Can you work these out from the model? Positions are in its coordinate system, mm. A direction names the side the tool comes from. Give positions to 0.01 mm unless a question says otherwise; leave off trailing zeros. Order: outer loops, then holes, each group sorted by start corner. A loop starts at its lowest first (then second) coordinate and runs counter-clockwise, first axis right, second up. Notation, with made-up numbers: (16, 46) - (29, 46) arc R18 ccw to (29, 74) - close; hole circle Ø7 at (78.5, -34). An arc over 180 degrees is marked (long way). Answer as CSV lines item,"result".
```python
from build123d import *

# Parameters (mm, degrees)
F1_DEPTH = 50
F2_R     = 15
F3_DEPTH = 90
F4_R     = 10
F5_R     = 5


with BuildPart() as f1:
    # F0 (on Top) → F1 (new body)
    with BuildSketch(Plane.XY):
        with BuildLine():
            Line((-53.892129, 40.60475), (-53.892129, -39.39525))
            Line((-53.892129, -39.39525), (-38.892129, -39.39525))
            Line((-38.892129, -39.39525), (-38.892129, 46.271418))
            Line((-38.892129, 46.271418), (28.441196, 46.271418))
            Line((28.441196, 46.271418), (28.441196, -39.39525))
            Line((28.441196, -39.39525), (43.441196, -39.39525))
            Line((43.441196, -39.39525), (43.441196, 40.60475))
            ThreePointArc((43.441196, 40.60475), (22.390443, 58.953554), (-4.5588, 66.271418))
            ThreePointArc((-4.5588, 66.271418), (-32.33335, 59.411682), (-53.892129, 40.60475))
        make_face()
    extrude(amount=F1_DEPTH)

    # F2 (on face) → F3 (cut)
    with BuildSketch(Plane.YZ.offset(43.441196)):
        with Locations((-17.843239, 25)):
            Circle(F2_R)
        with Locations((21.808403, 25)):
            Circle(F2_R)
    extrude(amount=-F3_DEPTH, mode=Mode.SUBTRACT)

    # F4
    f4_edges = [f1.edges().sort_by_distance(p)[0] for p in [
        (-46.392129, -39.39525, 50),
        (-46.392129, -39.39525, 0),
        (35.941196, -39.39525, 50),
        (35.941196, -39.39525, 0),
    ]]
    fillet(f4_edges, radius=F4_R)

    # F5
    f5_edges = [f1.edges().sort_by_distance(p)[0] for p in [
        (28.441196, 46.271418, 25),
        (-38.892129, 46.271418, 25),
    ]]
    fillet(f5_edges, radius=F5_R)


solid = f1.part
```
1) If we mould it in two halves opening along Z, with no side actions, what happens to faces 4 (the flat face through (-46.559, 22, 25)), 5 (the flat face through (13, 47, 50)), 6 (the cylindrical face through (-31.97, 59.6, 24.65)), 7 (the cylindrical face through (36.046, -36.388, 2.852))? For each: +Z half, -Z half, draft (parallel to the pull), parting line (faces both ways), or undercut.
Answer block:
face 4,"undercut"
face 5,"+Z half"
face 6,"draft"
face 7,"-Z half"
2) I'm going to push flat-ended pins straight in: P1, Ø24, axis at y = -17.84, z = 25, coming from the +X side; P2, Ø6, axis at x = 6, z = 44, coming from the -Y side; P3, Ø10, axis at x = -20, z = 44, coming from the +Y side; P4, Ø5, axis at x = 10.5, y = 43.5, coming from the +Z side. Where does each tip first touch, or does it pass through?
Answer block:
P1,"x = -46.56"
P2,"y = 46.27"
P3,"y = 65.32"
P4,"through"
3) I need wall thicknesses on line 1 along X through (y, z) = (-18, 9); line 2 along Y through (x, z) = (-5.5, 28); line 3 along X through (y, z) = (43, 16). Which ranges of each line are inside material? Lowest first, please. Write a range as [from, to].
Answer block:
line 1,"[-53.89, -38.89], [28.44, 43.44]"
line 2,"[46.27, 66.26]"
line 3,"[-52.11, -38.58], [28.13, 41.61]"
4) I want a section at D-D on z = 31. Write out the boundary of the cut face in (x, y), plus the area to 3 significant figures.
Answer block:
outline,"(-53.89, -39.4) - (-38.89, -39.4) - (-38.89, -31.59) - (-46.56, -31.59) - (-46.56, -4.1) - (-38.89, -4.1) - (-38.89, 8.06) - (-46.56, 8.06) - (-46.56, 35.56) - (-38.89, 35.56) - (-38.89, 41.27) arc R5 cw to (-33.89, 46.27) - (23.44, 46.27) arc R5 cw to (28.44, 41.27) - (28.44, 35.56) - (43.44, 35.56) - (43.44, 40.6) arc R62.34 ccw to (-4.56, 66.27) arc R60.77 ccw to (-53.89, 40.6) - close; (28.44, -39.4) - (43.44, -39.4) - (43.44, -31.59) - (28.44, -31.59) - close; (28.44, -4.1) - (43.44, -4.1) - (43.44, 8.06) - (28.44, 8.06) - close"
area,"2,510 mm2"
5) Which directions (+Z, -Z, +X, -X, +Y, -Y) give clear straight access to the entire face, cutting with the end or side of a thin tool? Please do faces 1 (the cylindrical face through (-37.466, 44.768, 25.35)), 2 (the flat face through (36, -39.395, 25)), 3 (the flat face through (-46.559, -18, 25)).
Answer block:
face 1,"+Z, -Z, -Y"
face 2,"+Z, -Z, +X, -X, -Y"
face 3,"+X"
6) I want a section at B-B on y = -9. Write out the boundary of the cut face in (x, z).
Answer block:
outline,"(-53.89, 0) - (-38.89, 0) - (-38.89, 12.88) - (-46.56, 12.88) - (-46.56, 37.12) - (-38.89, 37.12) - (-38.89, 50) - (-53.89, 50) - close; (28.44, 0) - (43.44, 0) - (43.44, 12.88) - (28.44, 12.88) - close; (28.44, 37.12) - (43.44, 37.12) - (43.44, 50) - (28.44, 50) - close"
7) I want a section at A-A on z = 25. Write out the boundary of the cut face in (x, y), plus the area to 3 significant figures.
Answer block:
outline,"(-53.89, -39.4) - (-38.89, -39.4) - (-38.89, -32.84) - (-46.56, -32.84) - (-46.56, -2.84) - (-38.89, -2.84) - (-38.89, 6.81) - (-46.56, 6.81) - (-46.56, 36.81) - (-38.89, 36.81) - (-38.89, 41.27) arc R5 cw to (-33.89, 46.27) - (23.44, 46.27) arc R5 cw to (28.44, 41.27) - (28.44, 36.81) - (43.44, 36.81) - (43.44, 40.6) arc R62.34 ccw to (-4.56, 66.27) arc R60.77 ccw to (-53.89, 40.6) - close; (28.44, -39.4) - (43.44, -39.4) - (43.44, -32.84) - (28.44, -32.84) - close; (28.44, -2.84) - (43.44, -2.84) - (43.44, 6.81) - (28.44, 6.81) - close"
area,"2,400 mm2"
8) I want a section at C-C on z = 5. Write out the boundary of the cut face in (x, y), plus the area to 3 significant figures.
Answer block:
outline,"(-53.89, -38.06) - (-38.89, -38.06) - (-38.89, 41.27) arc R5 cw to (-33.89, 46.27) - (23.44, 46.27) arc R5 cw to (28.44, 41.27) - (28.44, -38.06) - (43.44, -38.06) - (43.44, 40.6) arc R62.34 ccw to (-4.56, 66.27) arc R60.77 ccw to (-53.89, 40.6) - close"
area,"3,720 mm2"
